Autodesk Inventor part; units mm, degrees
ref_plane "YZ Plane" through (0, 0, 0) normal (1, 0, 0) x (0, 1, 0)
ref_plane "XZ Plane" through (0, 0, 0) normal (0, 1, 0) x (-1, 0, 0)
ref_plane "XY Plane" through (0, 0, 0) normal (0, 0, 1) x (1, 0, 0)
sketch "Sketch1" plane through (0, 0, 0) normal (0, 0, 1) x (1, 0, 0)
  circle A0 centre (0, 0) radius 19.05
  circle A1 centre (0, 63.5) radius 19.05
  line L0 (0, -78.74) -> (0, 116.84) construction
  circle A2 centre (0, 63.5) radius 25.4
  circle A3 centre (0, 0) radius 25.4
  arc A4 (-49.069, -13.148) -> (49.069, -13.148) centre (0, 0) ccw
  line L1 (0, 0) -> (49.069, -13.148) construction
  line L2 (0, 0) -> (50.8, 0) construction
  line L3 (0, 0) -> (-49.069, -13.148) construction
  line L4 (-49.069, -13.148) -> (-24.364, 70.6803)
  line L5 (49.069, -13.148) -> (24.364, 70.6803)
  dimension "crank_dia" = 38.1
  dimension "d2" = 38.1
  dimension "crank_ctc" = 63.5
  dimension "crank_wt" = 6.35
  dimension "d8" = 6.35
  dimension "crank_rad" = 50.8
  dimension "d10" = 15
  dimension "d13" = 150
extrude "Extrusion1" add sketch "Sketch1" along normal blind 9.525 contours A1
extrude "Extrusion2" add sketch "Sketch1" along normal blind 6.35 from surface at 9.525 contours A1 | A2 | A2 L5 A4 L4
extrude "Extrusion3" add sketch "Sketch1" along normal blind 76.2 from surface at 9.525 contours A0 | A3
mirror "Mirror1" about plane through (0, 0, 0) normal (0, 0, 1) of "Extrusion1", "Extrusion2", "Extrusion3"
equation "\"d2\" = 2 * pin_dia"
equation "\"d8\" = crank_wt"
properties part number "Crank_Shaft" material "Stainless Steel"
Verification items for the finished model (mm, model axes). A direction names the side the tool comes from. Round coordinates to 2 decimals unless told otherwise and drop trailing zeros. Order: outer loops, then holes, each group sorted by start corner. A loop starts at its lowest first (then second) coordinate and runs counter-clockwise, first axis right, second up. Notation, with made-up numbers: (29.5, 82.5) - (85.5, 82.5) arc R21 ccw to (85.5, 91.5) - close; hole circle Ø6 at (11, -39). An arc over 180 degrees is marked (long way). Use CSV: the item, a comma, the result in double quotes. Start each with the question number.
1) Section check C-C, the plane x = 0. Record the cut outline in (y, z) (3 decimals), plus the area to 3 significant figures.
2) Section check D-D, the plane z = 29. Record the cut outline in (x, y), plus the area to 3 significant figures.
3) Section check B-B, the plane y = 37. Record the cut outline in (x, z) (3 decimals).
4) Thickness scan on L1, parallel to Z at x = 18, y = 2 (3 decimals); L2, parallel to Z at x = 9, y = 40 (3 decimals); L3, parallel to Y at x = 19.5, z = 63.5. Record the ranges inside material, lowest first.
5) Mould release check, pull along Z, two halves, no side actions. Record for faces 4 (the flat face through (1, 36, -15.875)), 5 (the cylindrical face through (0.457, 88.896, -12.656)), 6 (the cylindrical face through (-4.13, 44.903, 0.133)): +Z half, -Z half, draft (parallel to the pull), parting line (faces both ways), or undercut.
6) Go/stop test with flat-tipped pins: P1, Ø1, axis at y = 12, z = 66.5, coming from the +X side; P2, Ø10, axis at y = -33, z = 6, coming from the +X side; P3, Ø6, axis at y = -6, z = 64.5, coming from the +X side; P4, Ø10, axis at x = -1.5, z = -16, coming from the -Y side. Record where each tip stops, or that it passes through.
7) Section check A-A, the plane x = 29. Record the cut outline in (y, z) (3 decimals).
8) Access from +Z, -Z, +X, -X, +Y, -Y to the whole of each face (thin tool, end or side, straight path). Record for faces 1 (the cylindrical face through (-0.93, -50.79, -12.66)), 2 (the cylindrical face through (-5.506, 24.796, 50.311)), 3 (the cylindrical face through (-5.506, -24.796, -50.311)).
Answers:
1,outline,"(-50.8, -15.875) - (-25.4, -15.875) - (-25.4, -85.725) - (25.4, -85.725) - (25.4, -15.875) - (88.9, -15.875) - (88.9, -9.525) - (82.55, -9.525) - (82.55, 9.525) - (88.9, 9.525) - (88.9, 15.875) - (25.4, 15.875) - (25.4, 85.725) - (-25.4, 85.725) - (-25.4, 15.875) - (-50.8, 15.875) - (-50.8, 9.525) - (44.45, 9.525) - (44.45, -9.525) - (-50.8, -9.525) - close"
1,area,"9,600 mm²"
2,outline,"circle Ø50.8 at (0, 0)"
2,area,"2,030 mm²"
3,outline,"(-34.29, -15.875) - (34.29, -15.875) - (34.29, -9.525) - (-34.29, -9.525) - close; (-34.29, 9.525) - (34.29, 9.525) - (34.29, 15.875) - (-34.29, 15.875) - close"
4,L1,"z = -85.725 to -9.525, 9.525 to 85.725"
4,L2,"z = -15.875 to -9.525, 9.525 to 15.875"
4,L3,"y = -16.28 to 16.28"
5,face 4,"-Z half"
5,face 5,"draft"
5,face 6,"undercut"
6,P1,"stops at x = 22.65"
6,P2,"stops at x = 41.39"
6,P3,"stops at x = 25.22"
6,P4,"stops at y = -50.8"
7,outline,"(-41.709, -15.875) - (54.95, -15.875) - (54.95, -9.525) - (-41.709, -9.525) - close; (-41.709, 9.525) - (54.95, 9.525) - (54.95, 15.875) - (-41.709, 15.875) - close"
8,face 1,"+Z, -Z, -Y"
8,face 2,"+Z"
8,face 3,"-Z"
